```python
from build123d import *

# Parameters (mm, degrees)
SKETCH1_R           = 3.275
BOSS_EXTRUDE1_DEPTH = 1
CHAMFER1_SIZE       = 0.2


with BuildPart() as part:
    # Sketch1 → Boss-Extrude1 (new body)
    with BuildSketch(Plane(origin=(0, 0, 0), x_dir=(1, 0, 0), z_dir=(0, 1, 0))):
        with BuildLine():
            Line((-9, 5.675), (9, 5.675))
            ThreePointArc((9, 5.675), (14.675, 0), (9, -5.675))
            Line((9, -5.675), (-9, -5.675))
            ThreePointArc((-9, -5.675), (-14.675, 0), (-9, 5.675))
        make_face()
        with Locations((-9, 0)):
            Circle(SKETCH1_R, mode=Mode.SUBTRACT)
        with Locations((9, 0)):
            Circle(SKETCH1_R, mode=Mode.SUBTRACT)
        with BuildLine():
            Line((-2.724651404, 3.275), (2.724651404, 3.275))
            ThreePointArc((2.724651404, 3.275), (3.543438303, 2.849097566), (3.664778535, 1.93417603))
            ThreePointArc((3.664778535, 1.93417603), (3.325, 0), (3.664778535, -1.93417603))
            ThreePointArc((3.664778535, -1.93417603), (3.543438303, -2.849097566), (2.724651404, -3.275))
            Line((2.724651404, -3.275), (-2.724651404, -3.275))
            ThreePointArc((-2.724651404, -3.275), (-3.543438303, -2.849097566), (-3.664778535, -1.93417603))
            ThreePointArc((-3.664778535, -1.93417603), (-3.325, 0), (-3.664778535, 1.93417603))
            ThreePointArc((-3.664778535, 1.93417603), (-3.543438303, 2.849097566), (-2.724651404, 3.275))
        make_face(mode=Mode.SUBTRACT)
    extrude(amount=BOSS_EXTRUDE1_DEPTH)

    # Chamfer1
    chamfer1_edges = [part.edges().sort_by_distance(p)[0] for p in [
        (-12.275, 0, 0),
        (-12.275, 1, 0),
        (14.675, 1, 0),
        (0, 1, -5.675),
        (3.543438303, 0, -2.849097566),
        (0, 0, -3.275),
        (-3.543438303, 0, -2.849097566),
        (-3.325, 0, 0),
        (-3.543438303, 0, 2.849097566),
        (0, 0, 3.275),
        (3.543438303, 0, 2.849097566),
        (3.325, 0, 0),
        (3.543438303, 1, -2.849097566),
        (0, 1, -3.275),
        (-3.543438303, 1, -2.849097566),
        (-3.325, 1, 0),
        (-3.543438303, 1, 2.849097566),
        (0, 1, 3.275),
        (3.543438303, 1, 2.849097566),
        (3.325, 1, 0),
        (5.725, 0, 0),
        (5.725, 1, 0),
        (-14.675, 1, 0),
        (0, 0, -5.675),
        (14.675, 0, 0),
        (0, 0, 5.675),
        (-14.675, 0, 0),
        (0, 1, 5.675),
    ]]
    chamfer(chamfer1_edges, length=CHAMFER1_SIZE)


solid = part.part
```
The listing builds one solid part. Answer for the finished solid, in the listing's coordinates (mm). A direction names the side the tool comes from. Coordinates: 2 decimals unless noted, no trailing zeros. Loops run counter-clockwise (first coordinate to the right, second up) from the corner with the lowest first, then second, coordinate; pieces in that order, holes last. Notation, with made-up numbers: (10, 27) -> (57, 27) arc R21 ccw to (57, 64) -> close; hole circle Ø5 at (42.5, 41). An arc over 180 degrees is marked (long way). Return JSON: item names as keys, results as strings. Group by question number.
(1) A cutting plane is placed at A-A on x = 2. Write down the section's boundary in (y, z) (3 decimals), and give its area (3 significant figures).
(2) Find the intervals of material crossed by probe 1 along Z at (x, y) = (-1.75, 0.75) (3 decimals); probe 2 along X at (y, z) = (0.1, -2); probe 3 along Z at (x, y) = (11.5, 0.3), in increasing order. Write a range as from..to.
(3) Given pin 1 Ø6 at (x, z) = (9, 0) entering from -Y, flat-ended and moving along its own axis, determine where the tip first touches the part or whether it passes through.
(4) Determine the mould class of faces 3 (the cylindrical face through (-14.674, 0.496, 0.125)), 4 (the flat face through (0, 0, 4)), 5 (the cylindrical face through (5.728, 0.496, -0.144)) for opening direction Z: released by +Z, released by -Z, zero draft, split by the parting line, or undercut.
(5) A cutting plane is placed at B-B on y = 0.4. Write down the section's boundary in (x, z) (3 decimals), and give its area (3 significant figures).
(6) Which of the six approach directions +Z, -Z, +X, -X, +Y, -Y give full straight-line access (tool end or side, diameter ignored) to faces 1 (the cylindrical face through (14.674, 0.496, -0.125)), 2 (the cylindrical face through (-3.536, 0.496, 2.86))?
(7) A cutting plane is placed at C-C on z = 0. Count the separate pieces of the cut face and the enclosed holes in it, and give its area (3 significant figures).
The answers:
{
 "1": {"outline": "(0, -5.475) -> (0.2, -5.675) -> (0.8, -5.675) -> (1, -5.475) -> (1, -3.475) -> (0.8, -3.275) -> (0.2, -3.275) -> (0, -3.475) -> close; (0, 3.475) -> (0.2, 3.275) -> (0.8, 3.275) -> (1, 3.475) -> (1, 5.475) -> (0.8, 5.675) -> (0.2, 5.675) -> (0, 5.475) -> close", "area": "4.64 mm^2"},
 "2": {"probe 1": "z = -5.675..-3.275, 3.275..5.675", "probe 2": "x = -14.2..-11.72, -6.28..-3.79, 3.79..6.28, 11.72..14.2", "probe 3": "z = -5.09..-2.12, 2.12..5.09"},
 "3": {"pin 1": "passes through"},
 "4": {"face 3": "split by the parting line", "face 4": "zero draft", "face 5": "undercut"},
 "5": {"outline": "(-9, -5.675) -> (9, -5.675) arc R5.675 ccw to (9, 5.675) -> (-9, 5.675) arc R5.675 ccw to start; hole circle Ø6.55 at (-9, 0); hole (-3.665, -1.934) arc R1 ccw to (-2.725, -3.275) -> (2.725, -3.275) arc R1 ccw to (3.665, -1.934) arc R5.675 cw to (3.665, 1.934) arc R1 ccw to (2.725, 3.275) -> (-2.725, 3.275) arc R1 ccw to (-3.665, 1.934) arc R5.675 cw to start; hole circle Ø6.55 at (9, 0)", "area": "192 mm^2"},
 "6": {"face 1": "+X, +Y, -Y", "face 2": "+Y, -Y"},
 "7": {"separate pieces": "4", "enclosed holes": "0", "area": "9.28 mm^2"}
}
